For this review, take the finished solid that the model builds, in its own axes (mm). Face numbers are marked on the shaded views. A direction names the side the tool comes from. Round coordinates to 2 decimals unless told otherwise and drop trailing zeros. Order: outer loops, then holes, each group sorted by start corner. A loop starts at its lowest first (then second) coordinate and runs counter-clockwise, first axis right, second up. Notation, with made-up numbers: M 47.25,67.5 L 100.25,67.5 A22 ccw 100.25,85.5 Z; hole C -31,-31.75 d10. An arc over 180 degrees is marked long. Answer as a JSON object with one key per item and string values.
Autodesk Inventor part; units mm, degrees
ref_plane "YZ Plane" through (0, 0, 0) normal (1, 0, 0) x (0, 1, 0)
ref_plane "XZ Plane" through (0, 0, 0) normal (0, 1, 0) x (-1, 0, 0)
ref_plane "XY Plane" through (0, 0, 0) normal (0, 0, 1) x (1, 0, 0)
sketch "Sketch1" plane through (0, 0, 0) normal (0, 0, 1) x (1, 0, 0)
  circle A0 centre (0, 0) radius 3
  line L0 (6, -4) -> (-6, -4)
  line L1 (-6, -4) -> (-6, 4)
  line L2 (-6, 4) -> (6, 4)
  line L3 (6, 4) -> (6, -4)
  line L4 (6, -4) -> (-6, 4) construction
  line L5 (-6, -4) -> (6, 4) construction
  line L6 (6, 4) -> (23.8, 4)
  line L7 (23.8, 4) -> (23.8, -4)
  line L8 (23.8, -4) -> (6, -4)
  line L9 (6, -4) -> (6, 4)
  point P0 (0, 0)
  dimension "d0" = 12
  dimension "d1" = 8
  dimension "d2" = 17.8
extrude "Extrusion1" add sketch "Sketch1" along normal blind 8
sketch "Sketch2" plane through (23.8, -4, 0) normal (1, 0, 0) x (0, 0, -1)
  circle A0 centre (-4, 4) radius 3
  point P0 (0, 4)
  dimension "d5" = 6
extrude "Extrusion2" cut sketch "Sketch2" against normal blind 19.8
sketch "Sketch3" plane through (-6, -4, 0) normal (-1, 0, 0) x (0, 0, 1)
  circle A0 centre (4, 4) radius 1.2
  point P0 (0, 4)
  dimension "d8" = 2.4
extrude "Extrusion3" cut sketch "Sketch3" against normal blind 4
thread "Thread1"
sketch "Sketch5" plane through (0, 0, 8) normal (0, 0, 1) x (1, 0, 0)
  line L0 (23.8, 4) -> (-6, 4)
  line L1 (-6, -4) -> (23.8, -4)
  line L2 (23.8, -4) -> (23.8, 4)
  line L3 (17.8, 4) -> (17.8, -4)
  dimension "d20" = 6
extrude "Extrusion5" add sketch "Sketch5" along normal blind 5.4
sketch "Sketch6" plane through (23.8, -4, 0) normal (1, 0, 0) x (0, 0, -1)
  line L0 (-13.4, 0) -> (-13.4, 8)
  circle A0 centre (-10.4, 4) radius 1.2
  point P0 (0, 4)
  dimension "d23" = 2.4
  dimension "d24" = 3
extrude "Extrusion6" cut sketch "Sketch6" against normal blind 10
thread "Thread3"
properties material "Copper"
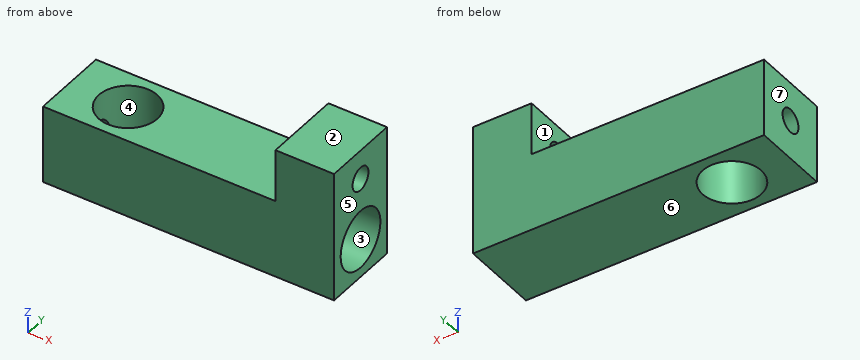
1) Machinability: for the marked faces 1, 2 and 3, which of the approach directions +Z, -Z, +X, -X, +Y, -Y give a long, thin tool a straight path to every point of the face, cutting with its end or side? Answer none if there is none.
Geometry check:
{"face 1": "+Z, -X, +Y, -Y", "face 2": "+Z, +X, -X, +Y, -Y", "face 3": "+X"}
2) Add section B-B on x = 0. State the section outline as (y, z) points, and give its area (3 significant figures).
Geometry check:
{"outline": "M -4,0 L -3,0 L -3,8 L -4,8 Z; M 3,0 L 4,0 L 4,8 L 3,8 Z", "area": "16.0 mm²"}
3) Add section D-D on y = -1.75. State the section outline as (x, z) points.
Geometry check:
{"outline": "M -6,0 L -2.44,0 L -2.44,8 L -6,8 Z; M 2.44,0 L 23.8,0 L 23.8,1.56 L 4,1.56 L 4,6.44 L 23.8,6.44 L 23.8,13.4 L 17.8,13.4 L 17.8,8 L 2.44,8 Z"}
4) Mouldability with a two-part tool opening along X and no side actions: class the marked faces 4, 5, 6 and 7 as +X half, -X half, draft (parallel to the pull), parting line (faces both ways), or undercut.
Geometry check:
{"face 4": "undercut", "face 5": "+X half", "face 6": "draft", "face 7": "-X half"}
5) Add section A-A on y = 0. State the section outline as (x, z) points, and give its area (3 significant figures).
Geometry check:
{"outline": "M -6,0 L -3,0 L -3,2.8 L -6,2.8 Z; M -6,5.2 L -3,5.2 L -3,8 L -6,8 Z; M 3,0 L 23.8,0 L 23.8,1 L 4,1 L 4,7 L 23.8,7 L 23.8,9.2 L 17.8,9.2 L 17.8,8 L 3,8 Z; M 17.8,11.6 L 23.8,11.6 L 23.8,13.4 L 17.8,13.4 Z", "area": "82.4 mm²"}
6) Add section C-C on z = 10.4. State the section outline as (x, y) points.
Geometry check:
{"outline": "M 17.8,-4 L 23.8,-4 L 23.8,-1.2 L 17.8,-1.2 Z; M 17.8,1.2 L 23.8,1.2 L 23.8,4 L 17.8,4 Z"}
7) Insertion check: P1, Ø4.5, axis at y = 1.5, z = 10.5, coming from the -X side; P2, Ø1.8, axis at y = 0.5, z = 5, coming from the +X side; P3, Ø2.5, axis at x = 1, y = 1.5, coming from the +Z side. Each pin has a flat end and moves straight along its axis. Give the tip position at first contact, or say it passes through.
Geometry check:
{"P1": "stops at x = 17.8", "P2": "stops at x = 4", "P3": "stops at z = 8"}
8) For L1, parallel to Y at x = 21.7, z = 10.4; L2, parallel to X at y = 0, z = 2.75; L3, parallel to X at y = -2.75, z = 6.75, list the stretches that pass through material, from the lowest coordinate up.
Geometry check:
{"L1": "y = -4 to -1.2, 1.2 to 4", "L2": "x = -6 to -3, 3 to 4", "L3": "x = -6 to -1.2, 1.2 to 23.8"}
